Could you check a few things on this model? Use its own coordinates, in mm. Face numbers are marked on the shaded views. A direction names the side the tool comes from. Coordinates: 2 decimals unless noted, no trailing zeros. Order: outer loops, then holes, each group sorted by start corner. A loop starts at its lowest first (then second) coordinate and runs counter-clockwise, first axis right, second up. Notation, with made-up numbers: (36.25, 22) -> (56.25, 22) arc R16 cw to (56.25, 49) -> close; hole circle Ø11 at (-18.75, -30). An arc over 180 degrees is marked (long way). Use a Markdown table: item, result. Add a question column.
1) If I drill on L1, parallel to X at y = 2, z = 0; L2, parallel to Y at x = 2, z = -2.5; L3, parallel to Y at x = -2.25, z = -1, over which ranges is the centre line in solid material (lowest first)? Write a range as [from, to].
2) If we section it at D-D (z = -1.5): Write out the boundary of the cut face in (x, y).
3) Thinking about a two-plate mould opening in X: for the marked faces 4, 5 and 6, which applies, +X half, -X half, draft (parallel to the pull), parting line (faces both ways), or undercut?
4) If we section it at B-B (x = 0): Write out the boundary of the cut face in (y, z), plus the area to 4 significant figures.
5) Will these pins go through, and if not, where does the flat tip stop? pin 1 Ø1.5 at (y, z) = (3.5, 1.5) entering from -X; pin 2 Ø3 at (x, z) = (0, 0) entering from +Y.
6) If we section it at A-A (z = 0): Write out the boundary of the cut face in (x, y), plus the area to 4 significant figures.
7) Which directions (+Z, -Z, +X, -X, +Y, -Y) give clear straight access to the entire face, cutting with the end or side of a thin tool? Please do the marked faces 1, 2 and 3.
8) If we section it at C-C (y = 0.35): Write out the boundary of the cut face in (x, z).
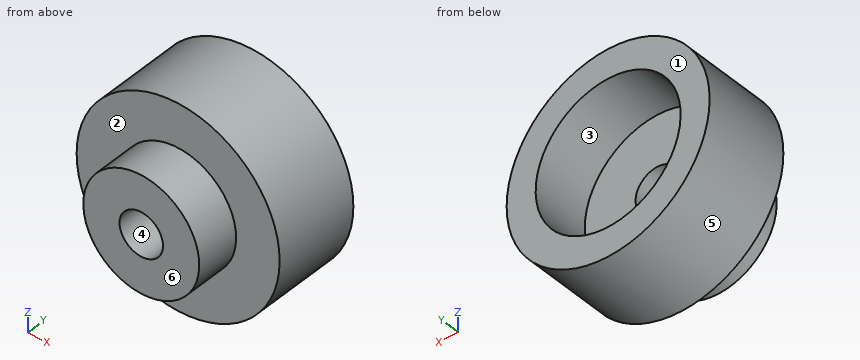
```python
from build123d import *

# Parameters (mm, degrees)
SKETCH1_R           = 1.5
SKETCH1_R_2         = 0.75
BOSS_EXTRUDE1_DEPTH = 2.5
SKETCH2_R           = 3.5
SKETCH2_R_2         = 2.5
BOSS_EXTRUDE2_DEPTH = 2
BOSS_EXTRUDE3_START = 1
SKETCH3_R           = 3.5
SKETCH3_R_2         = 0.75
BOSS_EXTRUDE3_DEPTH = 1
SKETCH4_R           = 2
SKETCH4_R_2         = 0.75
BOSS_EXTRUDE4_DEPTH = 2


with BuildPart() as part:
    # Sketch1 → Boss-Extrude1 (new body)
    with BuildSketch(Plane(origin=(0, 0, 0), x_dir=(1, 0, 0), z_dir=(0, 1, 0))):
        with Locations(Location((0, 0, 0), (0, 0, 270))):
            Circle(SKETCH1_R)
        with Locations(Location((0, 0, 0), (0, 0, 270))):
            Circle(SKETCH1_R_2, mode=Mode.SUBTRACT)
    extrude(amount=BOSS_EXTRUDE1_DEPTH)



with BuildPart() as body_2:
    # Sketch2 → Boss-Extrude2 (new body)
    with BuildSketch(Plane(origin=(0, 2.5, 0), x_dir=(1, 0, 0), z_dir=(0, 1, 0))):
        with Locations(Location((0, 0, 0), (0, 0, 270))):
            Circle(SKETCH2_R)
        with Locations(Location((0, 0, 0), (0, 0, 270))):
            Circle(SKETCH2_R_2, mode=Mode.SUBTRACT)
    extrude(amount=BOSS_EXTRUDE2_DEPTH)


with BuildPart() as part_1:
    add(part.part)

    add(body_2.part)  # Boss-Extrude3 merges body 2
    # Sketch3 → Boss-Extrude3 (add)
    with BuildSketch(Plane(origin=(0, 2.5, 0), x_dir=(-1, 0, 0), z_dir=(0, -1, 0)).offset(BOSS_EXTRUDE3_START)):
        with Locations(Location((0, 0, 0), (0, 0, 270))):
            Circle(SKETCH3_R)
        with Locations(Location((0, 0, 0), (0, 0, 270))):
            Circle(SKETCH3_R_2, mode=Mode.SUBTRACT)
    extrude(amount=-BOSS_EXTRUDE3_DEPTH)

    # Sketch4 → Boss-Extrude4 (add)
    with BuildSketch(Plane(origin=(0, 0, 0), x_dir=(-1, 0, 0), z_dir=(0, -1, 0))):
        with Locations(Location((0, 0, 0), (0, 0, 90))):
            Circle(SKETCH4_R)
        with Locations(Location((0, 0, 0), (0, 0, 270))):
            Circle(SKETCH4_R_2, mode=Mode.SUBTRACT)
    extrude(amount=-BOSS_EXTRUDE4_DEPTH)


solid = part_1.part
```
Answer sheet:
| question | item | result |
|---|---|---|
| 1 | L1 | [-3.5, -0.75], [0.75, 3.5] |
| 1 | L2 | [1.5, 4.5] |
| 1 | L3 | [1.5, 2.5] |
| 2 | outline | (-3.16, 1.5) -> (-1.32, 1.5) -> (-1.32, 0) -> (1.32, 0) -> (1.32, 1.5) -> (3.16, 1.5) -> (3.16, 4.5) -> (2, 4.5) -> (2, 2.5) -> (-2, 2.5) -> (-2, 4.5) -> (-3.16, 4.5) -> close |
| 3 | face 4 | undercut |
| 3 | face 5 | parting line |
| 3 | face 6 | draft |
| 4 | outline | (0, -2) -> (1.5, -2) -> (1.5, -3.5) -> (4.5, -3.5) -> (4.5, -2.5) -> (2.5, -2.5) -> (2.5, -0.75) -> (0, -0.75) -> close; (0, 0.75) -> (2.5, 0.75) -> (2.5, 2.5) -> (4.5, 2.5) -> (4.5, 3.5) -> (1.5, 3.5) -> (1.5, 2) -> (0, 2) -> close |
| 4 | area | 13.25 mm2 |
| 5 | pin 1 | x = -3.42 |
| 5 | pin 2 | y = 2.5 |
| 6 | outline | (-3.5, 1.5) -> (-2, 1.5) -> (-2, 0) -> (-0.75, 0) -> (-0.75, 2.5) -> (-2.5, 2.5) -> (-2.5, 4.5) -> (-3.5, 4.5) -> close; (0.75, 0) -> (2, 0) -> (2, 1.5) -> (3.5, 1.5) -> (3.5, 4.5) -> (2.5, 4.5) -> (2.5, 2.5) -> (0.75, 2.5) -> close |
| 6 | area | 13.25 mm2 |
| 7 | face 1 | +Z, -Z, +X, -X, +Y |
| 7 | face 2 | -Y |
| 7 | face 3 | +Y |
| 8 | outline | circle Ø4 at (0, 0); hole circle Ø1.5 at (0, 0) |
